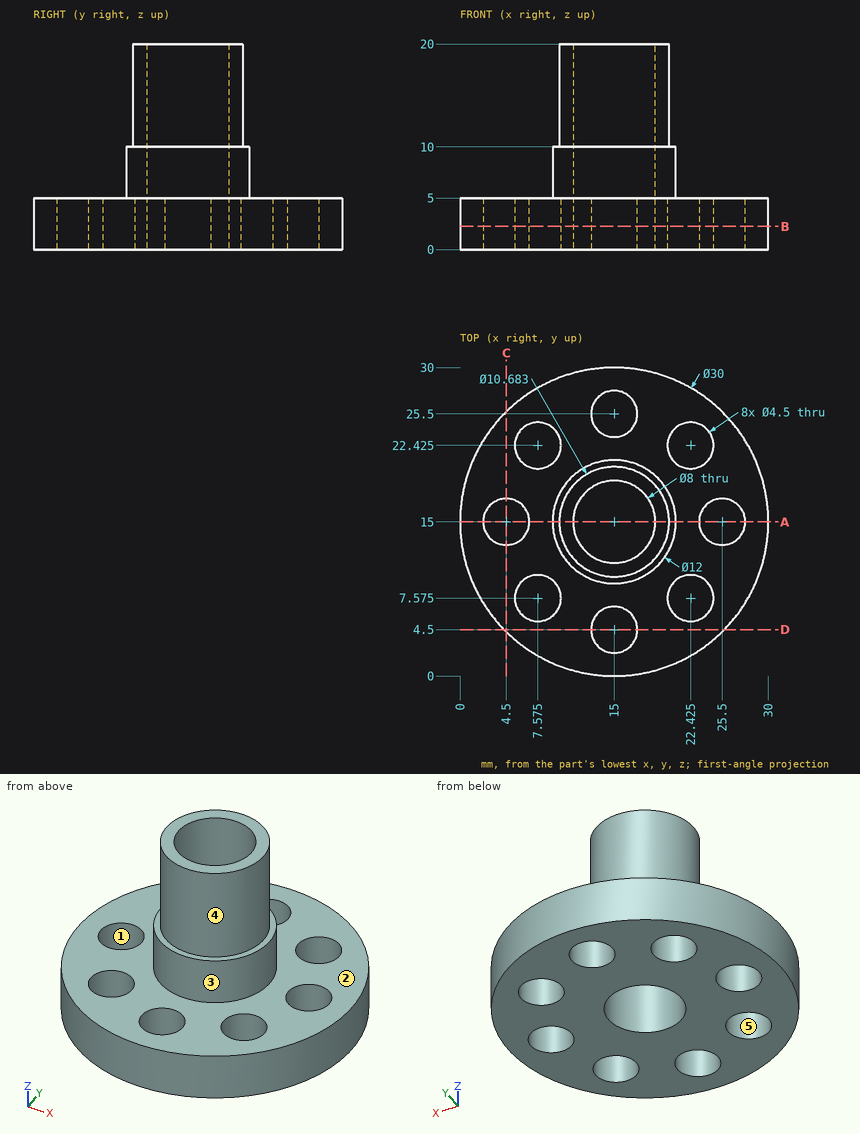
Here's the drawing with two shaded views (mm, measured from the low corner). I have some questions. A direction names the side the tool comes from. Coordinates: 2 decimals unless noted, no trailing zeros. Order: outer loops, then holes, each group sorted by start corner. A loop starts at its lowest first (then second) coordinate and runs counter-clockwise, first axis right, second up. Notation, with made-up numbers: (-8, 82.25) - (20, 82.25) arc R25 cw to (20, 114.25) - close; hole circle Ø2 at (-32.5, 32). An arc over 180 degrees is marked (long way). Answer in a Markdown table with one row per item. Add a question column.
(1) On a 3-axis mill with a long thin cutter (end or side, diameter ignored), from which of +Z, -Z, +X, -X, +Y, -Y can I reach the whole of each face in a straight line? I mean the marked faces 4 and 5. Say none if no direction works.
(2) I need wall thicknesses on L1, parallel to Y at x = 15, z = 9.5; L2, parallel to Y at x = 15.25, z = 14.25 (1 decimal); L3, parallel to Y at x = 15.5, z = 2.25. Which ranges of each line are inside material? Lowest first, please.
(3) Will these pins go through, and if not, where does the flat tip stop? pin 1 (6 mm diameter, centred on x = 15, y = 4.5, fed in from +Z); pin 2 (2 mm diameter, centred on x = 12, z = 16.5, fed in from +Y); pin 3 (7 mm diameter, centred on x = 15, y = 15, fed in from -Z); pin 4 (10 mm diameter, centred on y = 5, z = 11, fed in from +X).
(4) If we section it at B-B, the plane z = 2.25: State how many separate pieces and enclosed holes the cut face has.
(5) If we mould it in two halves opening along Y, with no side actions, what happens to the marked faces 1, 2 and 3? For each: released by +Y, released by -Y, zero draft, split by the parting line, or undercut.
(6) If we section it at A-A, the plane y = 15: Please give me the cut outline in (x, z), then the cut area to 3 significant figures.
(7) If we section it at C-C, the plane x = 4.5: Please give me the cut outline in (y, z).
Results are:
| question | item | result |
|---|---|---|
| 1 | face 4 | +Z |
| 1 | face 5 | +Z, -Z |
| 2 | L1 | y = 9 to 11, 19 to 21 |
| 2 | L2 | y = 9.7 to 11, 19 to 20.3 |
| 2 | L3 | y = 0.01 to 2.31, 6.69 to 11.03, 18.97 to 23.31, 27.69 to 29.99 |
| 3 | pin 1 | stops at z = 5 |
| 3 | pin 2 | stops at y = 19.95 |
| 3 | pin 3 | passes through |
| 3 | pin 4 | stops at x = 18.16 |
| 4 | separate pieces | 1 |
| 4 | enclosed holes | 9 |
| 5 | face 1 | undercut |
| 5 | face 2 | zero draft |
| 5 | face 3 | split by the parting line |
| 6 | outline | (0, 0) - (2.25, 0) - (2.25, 5) - (0, 5) - close; (6.75, 0) - (11, 0) - (11, 20) - (9.66, 20) - (9.66, 10) - (9, 10) - (9, 5) - (6.75, 5) - close; (19, 0) - (23.25, 0) - (23.25, 5) - (21, 5) - (21, 10) - (20.34, 10) - (20.34, 20) - (19, 20) - close; (27.75, 0) - (30, 0) - (30, 5) - (27.75, 5) - close |
| 6 | area | 112 mm2 |
| 7 | outline | (4.29, 0) - (12.75, 0) - (12.75, 5) - (4.29, 5) - close; (17.25, 0) - (25.71, 0) - (25.71, 5) - (17.25, 5) - close |
